Can you work these out from the model? Positions are in its coordinate system, mm. Face numbers are marked on the shaded views. A direction names the side the tool comes from. Coordinates: 2 decimals unless noted, no trailing zeros. Loops run counter-clockwise (first coordinate to the right, second up) from the corner with the lowest first, then second, coordinate; pieces in that order, holes last. Notation, with made-up numbers: (83, 80) -> (120, 80) arc R13 ccw to (120, 97) -> close; hole circle Ø9 at (80, 22.5). An arc over 180 degrees is marked (long way). Use one line per item in the form item = value. Start each with the question number.
(1) Imagine slicing it at B-B (y = 0.05). List the corners of the cut face in (x, z) for me (3 decimals).
(2) Imagine slicing it at C-C (x = -8.5). List the corners of the cut face in (y, z) for me (3 decimals).
(3) Imagine slicing it at A-A (z = 0.5). List the corners of the cut face in (x, y) for me (3 decimals).
(4) I need wall thicknesses on line 1 (X direction, y = 0.65, z = -3); line 2 (Y direction, x = 7, z = -2) (3 decimals); line 3 (Z direction, x = -6.25, y = -0.7) (3 decimals). Which ranges of each line are inside material? Lowest first, please. Write a range as [from, to].
(5) I'm going to push flat-ended pins straight in: pin 1 (1.3 mm diameter, centred on y = 0, z = 1.5, fed in from -X); pin 2 (1 mm diameter, centred on x = -6, z = -1.5, fed in from -Y) (3 decimals); pin 3 (1.1 mm diameter, centred on x = 6, y = 0, fed in from -Z) (3 decimals). Where does each tip first touch, or does it pass through?
(6) On a 3-axis mill with a long thin cutter (end or side, diameter ignored), from which of +Z, -Z, +X, -X, +Y, -Y can I reach the whole of each face in a straight line? I mean the marked faces 1, 2 and 3. Say none if no direction works.
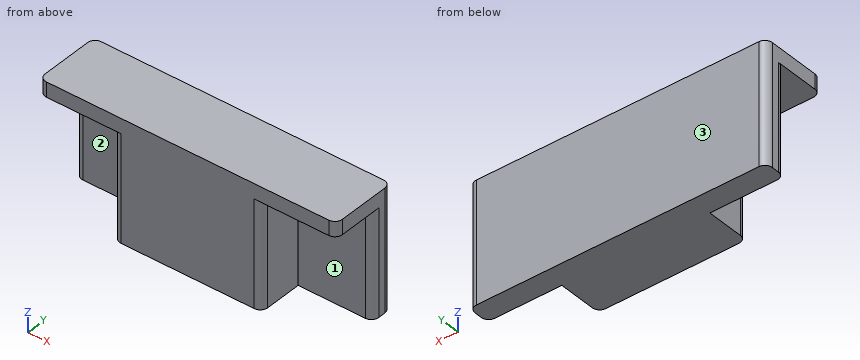
```python
from build123d import *

# Parameters (mm, degrees)
BOSS_EXTRUDE1_DEPTH = 3.575
SKETCH3_W           = 20
SKETCH3_H           = 4.51
BOSS_EXTRUDE2_DEPTH = 1
FILLET1_R           = 0.5


with BuildPart() as part:
    # Sketch2 → Boss-Extrude1 (new, symmetric)
    with BuildSketch(Plane.XY):
        Polygon((-4.98, -2.255), (4.98, -2.255), (4.98, 0.755), (10, 0.755), (10, 2.255), (-10, 2.255), (-10, 0.755), (-4.98, 0.755), align=None)
    extrude(amount=BOSS_EXTRUDE1_DEPTH, both=True)

    # Sketch3 → Boss-Extrude2 (add)
    with BuildSketch(Plane.XY.offset(3.575)):
        Rectangle(SKETCH3_W, SKETCH3_H)
    extrude(amount=BOSS_EXTRUDE2_DEPTH)

    # Fillet1
    fillet1_edges = [part.edges().sort_by_distance(p)[0] for p in [
        (-10, 0.755, 0),
        (-10, 2.255, 0.5),
        (10, 2.255, 0.5),
        (10, 0.755, 0),
        (4.98, -2.255, 0),
        (-4.98, -2.255, 0),
        (10, -2.255, 4.075),
        (-10, -2.255, 4.075),
    ]]
    fillet(fillet1_edges, radius=FILLET1_R)


solid = part.part
```
Worked out:
q1.outline = (-10, 3.575) -> (-4.98, 3.575) -> (-4.98, -3.575) -> (4.98, -3.575) -> (4.98, 3.575) -> (10, 3.575) -> (10, 4.575) -> (-10, 4.575) -> close
q2.outline = (-2.255, 3.575) -> (0.755, 3.575) -> (0.755, -3.575) -> (2.255, -3.575) -> (2.255, 4.575) -> (-2.255, 4.575) -> close
q3.outline = (-10, 1.255) arc R0.5 ccw to (-9.5, 0.755) -> (-4.98, 0.755) -> (-4.98, -1.755) arc R0.5 ccw to (-4.48, -2.255) -> (4.48, -2.255) arc R0.5 ccw to (4.98, -1.755) -> (4.98, 0.755) -> (9.5, 0.755) arc R0.5 ccw to (10, 1.255) -> (10, 1.755) arc R0.5 ccw to (9.5, 2.255) -> (-9.5, 2.255) arc R0.5 ccw to (-10, 1.755) -> close
q4.line_1 = [-4.98, 4.98]
q4.line_2 = [0.755, 2.255]
q4.line_3 = [3.575, 4.575]
q5.pin_1 = -4.98
q5.pin_2 = 0.755
q5.pin_3 = 3.575
q6.face_1 = -Z, +X, -Y
q6.face_2 = -Z, -X, -Y
q6.face_3 = +Z, -Z, +X, -X, +Y
